Here's how the part is built. I have some questions about the finished solid (model axes, mm). A direction names the side the tool comes from. Round coordinates to 2 decimals unless told otherwise and drop trailing zeros. Write each loop counter-clockwise with the first axis right and the second up, starting at its lowest first coordinate (ties: lowest second). Pieces come first, ordered by that corner, then holes. Notation, with made-up numbers: (-5.75, -8.75) - (16.25, -8.75) arc R24 ccw to (16.25, 7.25) - close; hole circle Ø5 at (-22.75, -3). An arc over 180 degrees is marked (long way). One line per question, with ' | ' between items. Start each with the question number.
(1) Imagine slicing it at C-C (x = -53). Write out the boundary of the cut face in (y, z), plus the area to 3 significant figures.
(2) Imagine slicing it at A-A (y = 37.5). Write out the boundary of the cut face in (x, z).
(3) Imagine slicing it at B-B (z = 4.75). Write out the boundary of the cut face in (x, y), plus the area to 3 significant figures.
(4) Will these pins go through, and if not, where does the flat tip stop? pin 1 (1 mm diameter, centred on x = -3.5, z = 7.5, fed in from +Y); pin 2 (2.5 mm diameter, centred on y = 28.5, z = 5, fed in from -X); pin 3 (5.5 mm diameter, centred on x = -18, y = -8.5, fed in from +Z).
(5) If I drill on L1, parallel to X at y = 54, z = 5.25; L2, parallel to Y at x = -76, z = 2.75; L3, parallel to Y at x = -31.5, z = 8.75, over which ranges is the centre line in solid material (lowest first)?
(6) For faces 4 (the cylindrical face through (26.049, 40.367, 3.972)), 5 (the flat face through (11, -8, 10)), 6 (the flat face through (-36.493, 21, 6)), 7 (the flat face through (0, 59.808, 5)), which set-ups out of +Z, -Z, +X, -X, +Y, -Y let a thin tool reach every point of the face, with its end or its side?
(7) Thinking about a two-plate mould opening in Y: for faces 1 (the cylindrical face through (9.815, -9.523, 7.972)), 2 (the flat face through (0, -23.192, 6)), 3 (the flat face through (32.507, 19, 6)), which applies, pulls with the +Y half, pulls with the -Y half, needs draft (parallel to the pull), parting line crosses it, or undercut?
Autodesk Fusion 360 part; units mm, degrees
sketch "Sketch1" plane through (0, 0, 0) normal (0, 0, 1) x (1, 0, 0)
  line L0 (-88.4927, 61.808) -> (34.5073, 61.808)
  line L1 (34.5073, 61.808) -> (34.5073, -25.192)
  line L2 (34.5073, -25.192) -> (-88.4927, -25.192)
  line L3 (-88.4927, -25.192) -> (-88.4927, 61.808)
  dimension "d1" = 123
  dimension "d2" = 87
extrude "Extrude1" add sketch "Sketch1" along normal blind 2
sketch "Sketch2" plane through (0, 0, 2) normal (0, 0, 1) x (-1, 0, 0)
  line L0 (88.4927, 25.192) -> (-34.5073, 25.192)
  line L1 (-34.5073, 25.192) -> (-34.5073, -61.808)
  line L2 (-34.5073, -61.808) -> (88.4927, -61.808)
  line L3 (88.4927, -61.808) -> (88.4927, 25.192)
  line L4 (88.4927, -61.808) -> (88.4927, -59.808)
  line L5 (88.4927, -61.808) -> (86.4927, -61.808)
  line L6 (86.4927, -61.808) -> (86.4927, -59.808)
  line L7 (86.4927, -59.808) -> (36.4927, -59.808)
  line L8 (88.4927, 25.192) -> (86.4927, 25.192)
  line L9 (86.4927, -59.808) -> (86.4927, 23.192)
  line L10 (86.4927, 23.192) -> (36.4927, 23.192)
  line L11 (86.4927, -59.808) -> (84.4927, -59.808)
  line L12 (36.4927, 23.192) -> (36.4927, 21.192)
  line L13 (36.4927, 21.192) -> (38.4927, 21.192)
  line L14 (84.4927, -57.808) -> (38.4927, -57.808)
  line L15 (38.4927, -57.808) -> (38.4927, 18.0206)
  line L16 (38.4927, 21.192) -> (84.4927, 21.192)
  line L17 (84.4927, 21.192) -> (84.4927, -57.808)
  line L18 (38.4927, 18.0206) -> (36.4927, 18.0206)
  line L19 (36.4927, -59.808) -> (36.4927, 18.0206)
  line L20 (36.4927, 21.192) -> (36.4927, 23.192)
  line L21 (-34.5073, 25.192) -> (-34.5073, 23.192)
  line L22 (-34.5073, 23.192) -> (-32.5073, 23.192)
  line L23 (-32.5073, -59.808) -> (-32.5073, 23.192)
  line L24 (-32.5073, 23.192) -> (32.4927, 23.192)
  line L25 (32.4927, -59.808) -> (30.4927, -59.808)
  line L26 (-32.5073, 23.192) -> (-32.5073, 21.192)
  line L27 (-30.5073, -57.808) -> (-30.5073, 21.192)
  line L28 (-30.5073, 21.192) -> (30.4927, 21.192)
  line L29 (30.4927, 18.0206) -> (30.4927, -57.808)
  line L30 (32.4927, 18.0206) -> (30.4927, 18.0206)
  line L31 (30.4927, 21.192) -> (32.4927, 21.192)
  line L32 (32.4927, 23.192) -> (32.4927, 21.192)
  line L33 (32.4927, 18.0206) -> (32.4927, -59.808)
  line L34 (30.4927, -59.808) -> (22.4927, -59.808)
  line L35 (12.4927, -59.808) -> (12.4927, -57.808)
  line L36 (22.4927, -57.808) -> (22.4927, -59.808)
  line L37 (30.4927, -57.808) -> (22.4927, -57.808)
  line L38 (32.4927, -59.808) -> (22.4927, -59.808)
  line L39 (12.4927, -59.808) -> (-32.5073, -59.808)
  line L40 (-32.5073, -59.808) -> (-15.5073, -59.808)
  line L41 (-5.5073, -59.808) -> (-5.5073, -57.808)
  line L42 (-5.5073, -57.808) -> (-15.5073, -57.808)
  line L43 (-15.5073, -57.808) -> (-15.5073, -59.808)
  line L44 (12.4927, -57.808) -> (-5.5073, -57.808)
  line L45 (-15.5073, -57.808) -> (-30.5073, -57.808)
  dimension "d5" = 2
  dimension "d6" = 2
  dimension "d7" = 2
  dimension "d8" = 50
  dimension "d9" = 2
  dimension "d10" = 2
  dimension "d11" = 50
  dimension "d12" = 2
  dimension "d13" = 2
  dimension "d14" = 2
  dimension "d15" = 2
  dimension "d17" = 4
  dimension "d18" = 2
  dimension "d19" = 2
  dimension "d20" = 2
  dimension "d21" = 2
  dimension "d22" = 2
  dimension "d23" = 2
  dimension "d24" = 8
  dimension "d25" = 10
  dimension "d26" = 17
  dimension "d27" = 10
extrude "Extrude2" add sketch "Sketch2" along normal blind 9 contours L23 L24 L26 L27 L28 L31 L32 L39 L40 L43 L45 | L7 L9 L10 L11 L12 L13 L14 L15 L16 L17 L18 L19 L20 | L35 L39 L41 L44 | L25 L29 L30 L33 L34 L36 L37 L38
sketch "Sketch3" plane through (0, 0, 2) normal (0, 0, 1) x (-1, 0, 0)
  line L0 (12.4927, -59.808) -> (-5.5073, -59.808)
  line L1 (-5.5073, -59.808) -> (-5.5073, -57.808)
  line L2 (-5.5073, -57.808) -> (12.4927, -57.808)
  line L3 (12.4927, -57.808) -> (12.4927, -59.808)
  line L4 (36.4927, 21.192) -> (36.4927, 23.192)
  line L5 (36.4927, 23.192) -> (86.4927, 23.192)
  line L6 (86.4927, 23.192) -> (86.4927, -59.808)
  line L7 (86.4927, -59.808) -> (36.4927, -59.808)
  line L8 (36.4927, -59.808) -> (36.4927, 18.0206)
  line L9 (36.4927, 18.0206) -> (38.4927, 18.0206)
  line L10 (38.4927, 18.0206) -> (38.4927, -57.808)
  line L11 (38.4927, -57.808) -> (84.4927, -57.808)
  line L12 (84.4927, -57.808) -> (84.4927, 21.192)
  line L13 (84.4927, 21.192) -> (36.4927, 21.192)
  line L14 (-32.5073, -59.808) -> (-32.5073, 23.192)
  line L15 (-32.5073, 23.192) -> (32.4927, 23.192)
  line L16 (32.4927, 23.192) -> (32.4927, 21.192)
  line L17 (32.4927, 21.192) -> (-30.5073, 21.192)
  line L18 (-30.5073, 21.192) -> (-30.5073, -57.808)
  line L19 (-30.5073, -57.808) -> (-15.5073, -57.808)
  line L20 (-15.5073, -57.808) -> (-15.5073, -59.808)
  line L21 (-15.5073, -59.808) -> (-32.5073, -59.808)
  line L22 (32.4927, 18.0206) -> (32.4927, -59.808)
  line L23 (32.4927, -59.808) -> (22.4927, -59.808)
  line L24 (22.4927, -59.808) -> (22.4927, -57.808)
  line L25 (22.4927, -57.808) -> (30.4927, -57.808)
  line L26 (30.4927, -57.808) -> (30.4927, 18.0206)
  line L27 (30.4927, 18.0206) -> (32.4927, 18.0206)
  line L28 (88.4927, 25.192) -> (-34.5073, 25.192)
  line L29 (-34.5073, 25.192) -> (-34.5073, -61.808)
  line L30 (-34.5073, -61.808) -> (88.4927, -61.808)
  line L31 (88.4927, -61.808) -> (88.4927, 25.192)
  line L32 (-5.5073, -59.808) -> (-15.5073, -59.808)
  line L33 (-15.5073, -59.808) -> (-15.5073, -57.808)
  line L34 (-15.5073, -57.808) -> (-5.5073, -57.808)
  line L35 (-5.5073, -57.808) -> (-5.5073, -59.808)
extrude "Extrude3" add sketch "Sketch3" along normal blind 4.5 contours L1 L20 L32 L33 L34 L35
sketch "Sketch4" plane through (0, 0, 2) normal (0, 0, 1) x (-1, 0, 0)
  line L0 (88.4927, 25.192) -> (-34.5073, 25.192)
  line L1 (-34.5073, 25.192) -> (-34.5073, -61.808)
  line L2 (-34.5073, -61.808) -> (88.4927, -61.808)
  line L3 (88.4927, -61.808) -> (88.4927, 25.192)
  line L4 (32.4927, 18.0206) -> (32.4927, -59.808)
  line L5 (32.4927, -59.808) -> (22.4927, -59.808)
  line L6 (22.4927, -59.808) -> (22.4927, -57.808)
  line L7 (22.4927, -57.808) -> (30.4927, -57.808)
  line L8 (30.4927, -57.808) -> (30.4927, 18.0206)
  line L9 (30.4927, 18.0206) -> (32.4927, 18.0206)
  line L10 (12.4927, -59.808) -> (-32.5073, -59.808)
  line L11 (-32.5073, -59.808) -> (-32.5073, 23.192)
  line L12 (-32.5073, 23.192) -> (32.4927, 23.192)
  line L13 (32.4927, 23.192) -> (32.4927, 21.192)
  line L14 (32.4927, 21.192) -> (-30.5073, 21.192)
  line L15 (-30.5073, 21.192) -> (-30.5073, -57.808)
  line L16 (-30.5073, -57.808) -> (12.4927, -57.808)
  line L17 (12.4927, -57.808) -> (12.4927, -59.808)
  line L18 (36.4927, 21.192) -> (36.4927, 23.192)
  line L19 (36.4927, 23.192) -> (86.4927, 23.192)
  line L20 (86.4927, 23.192) -> (86.4927, -59.808)
  line L21 (86.4927, -59.808) -> (36.4927, -59.808)
  line L22 (36.4927, -59.808) -> (36.4927, 18.0206)
  line L23 (36.4927, 18.0206) -> (38.4927, 18.0206)
  line L24 (38.4927, 18.0206) -> (38.4927, -57.808)
  line L25 (38.4927, -57.808) -> (84.4927, -57.808)
  line L26 (84.4927, -57.808) -> (84.4927, 21.192)
  line L27 (84.4927, 21.192) -> (36.4927, 21.192)
  circle A0 centre (23.9927, -42.808) radius 2.5
  circle A1 centre (-25.5073, -42.808) radius 2.5
  circle A2 centre (-10.5073, 8.192) radius 2.5
  circle A3 centre (18.4927, 8.192) radius 2.5
  dimension "d34" = 5
  dimension "d36" = 5
  dimension "d39" = 5
  dimension "d41" = 5
extrude "Extrude4" add sketch "Sketch4" along normal blind 4 contours A0 | A1 | A2 | A3
sketch "Sketch5" plane through (0, 0, 6) normal (0, 0, 1) x (-1, 0, 0)
  circle A0 centre (23.9927, -42.808) radius 2.5
  circle A1 centre (23.9927, -42.808) radius 1.5
  dimension "d44" = 3
extrude "Extrude5" add sketch "Sketch5" along normal blind 4 contours A1
sketch "Sketch6" plane through (0, 0, 6) normal (0, 0, 1) x (-1, 0, 0)
  circle A0 centre (-25.5073, -42.808) radius 2.5
  circle A1 centre (-25.5073, -42.808) radius 1.5
  dimension "d47" = 3
extrude "Extrude6" add sketch "Sketch6" along normal blind 4 contours A1
sketch "Sketch7" plane through (0, 0, 6) normal (0, 0, 1) x (-1, 0, 0)
  circle A0 centre (18.4927, 8.192) radius 2.5
  circle A1 centre (18.4927, 8.192) radius 1.5
  dimension "d50" = 3
extrude "Extrude7" add sketch "Sketch7" along normal blind 4 contours A1
sketch "Sketch8" plane through (0, 0, 6) normal (0, 0, 1) x (-1, 0, 0)
  circle A0 centre (-10.5073, 8.192) radius 2.5
  circle A1 centre (-10.5073, 8.192) radius 1.5
  dimension "d53" = 3
extrude "Extrude8" add sketch "Sketch8" along normal blind 4 contours A1
sketch "Sketch9" plane through (0, 0, 2) normal (0, 0, 1) x (-1, 0, 0)
  circle A0 centre (18.4927, 8.192) radius 2.5
  circle A1 centre (23.9927, -42.808) radius 2.5
  circle A2 centre (-10.5073, 8.192) radius 2.5
  circle A3 centre (-25.5073, -42.808) radius 2.5
  line L0 (88.4927, 25.192) -> (-34.5073, 25.192)
  line L1 (-34.5073, 25.192) -> (-34.5073, -61.808)
  line L2 (-34.5073, -61.808) -> (88.4927, -61.808)
  line L3 (88.4927, -61.808) -> (88.4927, 25.192)
  line L4 (32.4927, 18.0206) -> (32.4927, -59.808)
  line L5 (32.4927, -59.808) -> (22.4927, -59.808)
  line L6 (22.4927, -59.808) -> (22.4927, -57.808)
  line L7 (22.4927, -57.808) -> (30.4927, -57.808)
  line L8 (30.4927, -57.808) -> (30.4927, 18.0206)
  line L9 (30.4927, 18.0206) -> (32.4927, 18.0206)
  line L10 (12.4927, -59.808) -> (-32.5073, -59.808)
  line L11 (-32.5073, -59.808) -> (-32.5073, 23.192)
  line L12 (-32.5073, 23.192) -> (32.4927, 23.192)
  line L13 (32.4927, 23.192) -> (32.4927, 21.192)
  line L14 (32.4927, 21.192) -> (-30.5073, 21.192)
  line L15 (-30.5073, 21.192) -> (-30.5073, -57.808)
  line L16 (-30.5073, -57.808) -> (12.4927, -57.808)
  line L17 (12.4927, -57.808) -> (12.4927, -59.808)
  line L18 (36.4927, 21.192) -> (36.4927, 23.192)
  line L19 (36.4927, 23.192) -> (86.4927, 23.192)
  line L20 (86.4927, 23.192) -> (86.4927, -59.808)
  line L21 (86.4927, -59.808) -> (36.4927, -59.808)
  line L22 (36.4927, -59.808) -> (36.4927, 18.0206)
  line L23 (36.4927, 18.0206) -> (38.4927, 18.0206)
  line L24 (38.4927, 18.0206) -> (38.4927, -57.808)
  line L25 (38.4927, -57.808) -> (84.4927, -57.808)
  line L26 (84.4927, -57.808) -> (84.4927, 21.192)
  line L27 (84.4927, 21.192) -> (36.4927, 21.192)
  line L28 (22.4927, -59.808) -> (12.4927, -59.808)
  line L29 (12.4927, -59.808) -> (12.4927, -57.808)
  line L30 (12.4927, -57.808) -> (22.4927, -57.808)
  line L31 (22.4927, -57.808) -> (22.4927, -59.808)
extrude "Extrude9" add sketch "Sketch9" along normal blind 4.5 contours L6 L17 L28 L29 L30 L31
Check sheet entries:
1) outline: (-25.19, 0) - (61.81, 0) - (61.81, 2) - (59.81, 2) - (59.81, 11) - (57.81, 11) - (57.81, 2) - (-21.19, 2) - (-21.19, 11) - (-23.19, 11) - (-23.19, 2) - (-25.19, 2) - close | area: 210 mm^2
2) outline: (-88.49, 0) - (34.51, 0) - (34.51, 2) - (32.51, 2) - (32.51, 11) - (30.51, 11) - (30.51, 2) - (-30.49, 2) - (-30.49, 11) - (-32.49, 11) - (-32.49, 2) - (-36.49, 2) - (-36.49, 11) - (-38.49, 11) - (-38.49, 2) - (-84.49, 2) - (-84.49, 11) - (-86.49, 11) - (-86.49, 2) - (-88.49, 2) - close
3) outline: (-86.49, -23.19) - (-36.49, -23.19) - (-36.49, -21.19) - (-84.49, -21.19) - (-84.49, 57.81) - (-38.49, 57.81) - (-38.49, -18.02) - (-36.49, -18.02) - (-36.49, 59.81) - (-86.49, 59.81) - close; (-32.49, -23.19) - (32.51, -23.19) - (32.51, 59.81) - (-32.49, 59.81) - (-32.49, -18.02) - (-30.49, -18.02) - (-30.49, 57.81) - (30.51, 57.81) - (30.51, -21.19) - (-32.49, -21.19) - close; circle Ø5 at (-23.99, 42.81); circle Ø5 at (-18.49, -8.19); circle Ø5 at (10.51, -8.19); circle Ø5 at (25.51, 42.81) | area: 1,160 mm^2
4) pin 1: y = 59.81 | pin 2: x = -86.49 | pin 3: z = 10
5) L1: -86.49 to -84.49, -38.49 to -36.49, -32.49 to -30.49, 30.51 to 32.51 | L2: -23.19 to -21.19, 57.81 to 59.81 | L3: -23.19 to -21.19, -18.02 to 59.81
6) face 4: +Z | face 5: +Z, +Y | face 6: +Z, +Y, -Y | face 7: +Z, +X, -X, +Y
7) face 1: undercut | face 2: pulls with the -Y half | face 3: needs draft
